Build history of the part. All positions in model axes, mm. A direction names the side the tool comes from. Coordinates: 2 decimals unless noted, no trailing zeros. Order: outer loops, then holes, each group sorted by start corner. A loop starts at its lowest first (then second) coordinate and runs counter-clockwise, first axis right, second up. Notation, with made-up numbers: (-8.75, -28.75) - (15.25, -28.75) arc R6 ccw to (15.25, -23.75) - close; hole circle Ø9 at (60.25, 1). An arc over 180 degrees is marked (long way). Return JSON: item names as keys, results as strings.
from build123d import *

# Parameters (mm, degrees)
F0_W     = 6.35
F0_H     = 38.1
F1_DEPTH = 152.4


with BuildPart() as f1:
    # F0 (on Right) → F1 (new body, symmetric)
    with BuildSketch(Plane.YZ):
        Polygon((-11.1125, 25.4), (-20.6375, 25.4), (-20.6375, -25.4), (-11.1125, -25.4), (-11.1125, -19.05), (-11.1125, 19.05), align=None)
        with Locations((-7.9375, 0)):
            Rectangle(F0_W, F0_H)
    extrude(amount=F1_DEPTH, both=True)


solid = f1.part
1. Cut at A-A on x = -33.5. Give the cut face in (y, z), plus the area to 3 significant figures.
Check values:
{"outline": "(-20.64, -25.4) - (-11.11, -25.4) - (-11.11, -19.05) - (-4.76, -19.05) - (-4.76, 19.05) - (-11.11, 19.05) - (-11.11, 25.4) - (-20.64, 25.4) - close", "area": "726 mm²"}
2. Cut at C-C on z = 22. Give the cut face in (x, y).
Check values:
{"outline": "(-152.4, -20.64) - (152.4, -20.64) - (152.4, -11.11) - (-152.4, -11.11) - close"}
3. Drop flat-ended pins along their axis: pin 1 (7 mm diameter, centred on x = 49, y = -7.5, fed in from +Z); pin 2 (1.9 mm diameter, centred on x = 0, y = -6.5, fed in from -Z). Give the stop position or say it passes through.
Check values:
{"pin 1": "z = 19.05", "pin 2": "z = -19.05"}
4. Probe L1, parallel to Z at x = 98, y = -6.75; L2, parallel to Y at x = 110, z = -20. List the from-to ranges inside material, lowest first.
Check values:
{"L1": "-19.05 to 19.05", "L2": "-20.64 to -11.11"}
5. Tool access for faces 1 (the flat face through (2, -8, 19.05)), 2 (the flat face through (-152.4, -13, 0)), 3 (the flat face through (2, -11.112, -22)): list every direction of +Z, -Z, +X, -X, +Y, -Y with a clear straight run to the whole face (end or side of a thin tool).
Check values:
{"face 1": "+Z, +X, -X, +Y", "face 2": "+Z, -Z, -X, +Y, -Y", "face 3": "-Z, +X, -X, +Y"}
6. Cut at B-B on y = -8.5. Give the cut face in (x, z).
Check values:
{"outline": "(-152.4, -19.05) - (152.4, -19.05) - (152.4, 19.05) - (-152.4, 19.05) - close"}
